from build123d import *

# Parameters (mm, degrees)
SKETCH2_W           = 12
SKETCH2_H           = 18
BOSS_EXTRUDE1_DEPTH = 15
SKETCH5_R           = 3.5
CUT_EXTRUDE2_DEPTH  = 18
SKETCH8_W           = 3.937037176
SKETCH8_H           = 14
CUT_EXTRUDE3_DEPTH  = 1.492750999
FILLET3_R           = 0.05
SKETCH10_R          = 1.05
CUT_EXTRUDE6_DEPTH  = 3
FILLET9_R           = 0.5
FILLET10_R          = 0.5


with BuildPart() as part:
    # Sketch2 → Boss-Extrude1 (new body)
    with BuildSketch(Plane.XY):
        Rectangle(SKETCH2_W, SKETCH2_H)
    extrude(amount=BOSS_EXTRUDE1_DEPTH)

    # Sketch5 → Cut-Extrude2 (cut)
    with BuildSketch(Plane(origin=(0, -9, 0), x_dir=(-1, 0, 0), z_dir=(0, -1, 0))):
        with Locations((0, -7.5)):
            Circle(SKETCH5_R)
    extrude(amount=-CUT_EXTRUDE2_DEPTH, mode=Mode.SUBTRACT)

    # Sketch8 → Cut-Extrude3 (cut)
    with BuildSketch(Plane.XY.offset(15)):
        with Locations((0, 0.05)):
            Rectangle(SKETCH8_W, SKETCH8_H)
    extrude(amount=-CUT_EXTRUDE3_DEPTH, mode=Mode.SUBTRACT)

    # Fillet3
    fillet3_edges = [part.edges().sort_by_distance(p)[0] for p in [
        (-6, 0, 15),
        (0, -9, 15),
        (6, 0, 15),
        (0, -9, 0),
        (-6, 0, 0),
        (0, 9, 0),
        (6, 0, 0),
        (0, 9, 15),
        (6, -9, 7.5),
        (-6, -9, 7.5),
        (-6, 9, 7.5),
        (6, 9, 7.5),
    ]]
    fillet(fillet3_edges, radius=FILLET3_R)

    # Sketch10 → Cut-Extrude6 (cut)
    with BuildSketch(Plane.XY.offset(13.507249001)):
        with Locations((-0.031481412, 3.55)):
            Circle(SKETCH10_R)
        with Locations((-0.031481412, -5)):
            Circle(SKETCH10_R)
    extrude(amount=-CUT_EXTRUDE6_DEPTH, mode=Mode.SUBTRACT)

    # Fillet9
    fillet9_edges = [part.edges().sort_by_distance(p)[0] for p in [
        (-1.968518588, 0.05, 15),
        (0, -6.95, 15),
        (1.968518588, 0.05, 15),
        (0, 7.05, 15),
    ]]
    fillet(fillet9_edges, radius=FILLET9_R)

    # Fillet10
    fillet10_edges = [part.edges().sort_by_distance(p)[0] for p in [
        (-1.968518588, 0.05, 13.507249001),
        (0, 7.05, 13.507249001),
        (1.968518588, 0.05, 13.507249001),
        (0, -6.95, 13.507249001),
    ]]
    fillet(fillet10_edges, radius=FILLET10_R)


solid = part.part
Geometry check sheet. Reference: the model listing, model coordinates, mm. A direction names the side the tool comes from. Give positions to 0.01 mm unless a question says otherwise; leave off trailing zeros. Write each loop counter-clockwise with the first axis right and the second up, starting at its lowest first coordinate (ties: lowest second). Pieces come first, ordered by that corner, then holes. Notation, with made-up numbers: M 29.25,-0.75 L 65.25,-0.75 A17 cw 65.25,23.25 Z; hole C 89.5,71 d8. An arc over 180 degrees is marked long. Answer as CSV lines item,"result". Start each with the question number.
Q1. Tool access check on faces 1 (the face through (-1.88, -0.13, 4.55)), 2 (the face through (-0.259, 2.525, 12.184)). Record the directions out of +Z, -Z, +X, -X, +Y, -Y that give a thin tool (end or side, any length) a straight path to the whole face; none if there is none.
Q2. Section check A-A, the plane z = 7.5. Record the cut outline in (x, y).
Q3. Section check D-D, the plane z = 14.25. Record the cut outline in (x, y).
Q4. Section check C-C, the plane x = 0. Record the cut outline in (y, z).
Q5. Section check B-B, the plane y = -1.75. Record the cut outline in (x, z), then the cut area to 3 significant figures.
Q6. Material ranges on L1, parallel to X at y = -6, z = 14.25; L2, parallel to Z at x = 0, y = -2; L3, parallel to X at y = -0.5, z = 7.5, recorded low to high.
Q7. Go/stop test with flat-tipped pins: pin 1 (1.5 mm diameter, centred on x = 0, y = -1.5, fed in from +Z); pin 2 (1.3 mm diameter, centred on x = -0.03, y = -5, fed in from +Z); pin 3 (5 mm diameter, centred on x = 1, y = -5.5, fed in from +Z); pin 4 (3.5 mm diameter, centred on x = -0.03, y = 3.55, fed in from +Z). Record where each tip stops, or that it passes through.
Q8. Release check for a two-part mould opening along X. For faces 3 (the face through (-0.259, -6.025, 12.184)), 4 (the face through (-6, 0, 7)), 5 (the face through (0, 0, 13.507)), 6 (the face through (-1.4, -9, 4.1)) record: pulls with the +X half, pulls with the -X half, needs draft (parallel to the pull), parting line crosses it, or undercut.
Geometry says:
1,face 1,"+Y, -Y"
1,face 2,"+Z"
2,outline,"M -6,-8.95 A0.05 ccw -5.95,-9 L -3.5,-9 L -3.5,9 L -5.95,9 A0.05 ccw -6,8.95 Z; M 3.5,-9 L 5.95,-9 A0.05 ccw 6,-8.95 L 6,8.95 A0.05 ccw 5.95,9 L 3.5,9 Z"
3,outline,"M -6,-8.95 A0.05 ccw -5.95,-9 L 5.95,-9 A0.05 ccw 6,-8.95 L 6,8.95 A0.05 ccw 5.95,9 L -5.95,9 A0.05 ccw -6,8.95 Z; hole M -1.97,-6.95 L 1.97,-6.95 L 1.97,7.05 L -1.97,7.05 Z"
4,outline,"M -9,0.05 A0.05 ccw -8.95,0 L 8.95,0 A0.05 ccw 9,0.05 L 9,4 L -9,4 Z; M -9,11 L -6.05,11 L -6.05,13.51 L -6.45,13.51 A0.5 cw -6.95,14.01 L -6.95,14.5 A0.5 ccw -7.45,15 L -8.95,15 A0.05 ccw -9,14.95 Z; M -3.95,11 L 2.5,11 L 2.5,13.51 L -3.95,13.51 Z; M 4.6,11 L 9,11 L 9,14.95 A0.05 ccw 8.95,15 L 7.55,15 A0.5 ccw 7.05,14.5 L 7.05,14.01 A0.5 cw 6.55,13.51 L 4.6,13.51 Z"
5,outline,"M -6,0.05 A0.05 ccw -5.95,0 L 5.95,0 A0.05 ccw 6,0.05 L 6,14.95 A0.05 ccw 5.95,15 L 2.47,15 A0.5 ccw 1.97,14.5 L 1.97,14.01 A0.5 cw 1.47,13.51 L -1.47,13.51 A0.5 cw -1.97,14.01 L -1.97,14.5 A0.5 ccw -2.47,15 L -5.95,15 A0.05 ccw -6,14.95 Z; hole C 0,7.5 d7"
5,area,"136 mm^2"
6,L1,"-6 to -1.97, 1.97 to 6"
6,L2,"0 to 4, 11 to 13.51"
6,L3,"-6 to -3.5, 3.5 to 6"
7,pin 1,"z = 13.51"
7,pin 2,"z = 4.07"
7,pin 3,"z = 15"
7,pin 4,"z = 13.62"
8,face 3,"undercut"
8,face 4,"pulls with the -X half"
8,face 5,"undercut"
8,face 6,"needs draft"
